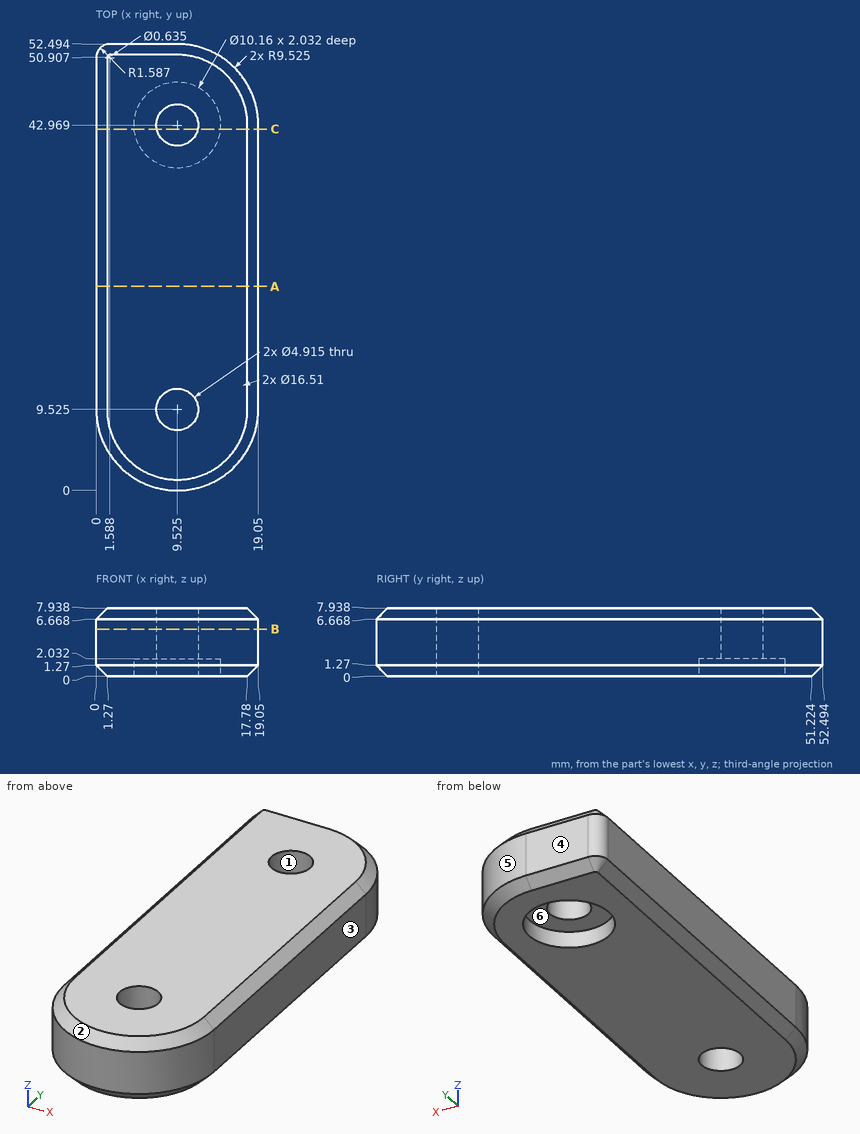
Drawing for the job (mm, zero at the part's lowest x, y, z). A direction names the side the tool comes from. Round coordinates to 2 decimals unless told otherwise and drop trailing zeros. Order: outer loops, then holes, each group sorted by start corner. A loop starts at its lowest first (then second) coordinate and runs counter-clockwise, first axis right, second up.
Item 1: Probe line 1 along Y through (x, z) = (9.75, 6); line 2 along Y through (x, z) = (11.75, 0.5) (1 decimal); line 3 along Z through (x, y) = (11.5, 39). List the from-to ranges inside material, lowest first.
Item 2: Pin check, flat tips, straight feed: pin 1 (5 mm diameter, centred on x = 9.5, y = 43.5, fed in from -Z); pin 2 (4.5 mm diameter, centred on x = 9.53, y = 42.97, fed in from -Z); pin 3 (3 mm diameter, centred on x = 7, z = 7, fed in from -Y). Stop position of each tip, or through.
Item 3: Tool access for the marked faces 5 and 6: list every direction of +Z, -Z, +X, -X, +Y, -Y with a clear straight run to the whole face (end or side of a thin tool).
Item 4: Saw through at A-A on y = 24. Write the cut outline in (x, z).
Item 5: Saw through at C-C on y = 42.5. Write the cut outline in (x, z).
Item 6: Saw through at B-B on z = 5.5. State how many separate pieces and enclosed holes the cut face has, then the cut area to 3 significant figures.
Item 7: Mould opens along Y. For the marked faces 1, 2, 3 and 4 say: pulls with the +Y half, pulls with the -Y half, needs draft (parallel to the pull), parting line crosses it, or undercut.
Reported:
1. line 1: y = 0 to 7.08, 11.97 to 40.52, 45.42 to 52.49
1. line 2: y = 1.1 to 8.5, 10.6 to 38.4, 47.5 to 51.4
1. line 3: z = 2.03 to 7.94
2. pin 1: stops at z = 2.03
2. pin 2: passes through
2. pin 3: stops at y = 0.06
3. face 5: +Z, -Z, +X, +Y
3. face 6: -Z
4. outline: (0, 1.27) - (1.27, 0) - (17.78, 0) - (19.05, 1.27) - (19.05, 6.67) - (17.78, 7.94) - (1.27, 7.94) - (0, 6.67) - close
5. outline: (0, 1.27) - (1.27, 0) - (4.47, 0) - (4.47, 2.03) - (7.11, 2.03) - (7.11, 7.94) - (1.27, 7.94) - (0, 6.67) - close; (11.94, 2.03) - (14.58, 2.03) - (14.58, 0) - (17.78, 0) - (19.05, 1.27) - (19.05, 6.67) - (17.78, 7.94) - (11.94, 7.94) - close
6. separate pieces: 1
6. enclosed holes: 2
6. area: 903 mm2
7. face 1: undercut
7. face 2: pulls with the -Y half
7. face 3: needs draft
7. face 4: pulls with the +Y half
